from build123d import *

# Parameters (mm, degrees)
F1_DEPTH = 130
F3_DEPTH = 600


with BuildPart() as f1:
    # F0 (on Front) → F1 (new body, symmetric)
    with BuildSketch(Plane.XZ):
        with BuildLine():
            Line((-250.1273464697, -45), (-246.1273464697, -45))
            Line((-246.1273464697, -45), (-246.1273464697, 0))
            ThreePointArc((-246.1273464697, 0), (-241.7339481875, 10.6066017178), (-231.1273464697, 15))
            Line((-231.1273464697, 15), (298.8726535303, 15))
            ThreePointArc((298.8726535303, 15), (309.4792552481, 10.6066017178), (313.8726535303, 0))
            Line((313.8726535303, 0), (313.8726535303, -45))
            Line((313.8726535303, -45), (317.8726535303, -45))
            Line((317.8726535303, -45), (317.8726535303, 0))
            ThreePointArc((317.8726535303, 0), (312.3076823729, 13.4350288425), (298.8726535303, 19))
            Line((298.8726535303, 19), (-231.1273464697, 19))
            ThreePointArc((-231.1273464697, 19), (-244.5623753122, 13.4350288425), (-250.1273464697, 0))
            Line((-250.1273464697, 0), (-250.1273464697, -45))
        make_face()
    extrude(amount=F1_DEPTH, both=True)

    # F2 (on face) → F3 (cut)
    with BuildSketch(Plane.YZ.offset(317.8726535303)):
        with BuildLine():
            Line((-70, -45), (70, -45))
            Line((70, -45), (70, -40))
            ThreePointArc((70, -40), (68.5355339059, -36.4644660941), (65, -35))
            Line((65, -35), (-65, -35))
            ThreePointArc((-65, -35), (-68.5355339059, -36.4644660941), (-70, -40))
            Line((-70, -40), (-70, -45))
        make_face()
    extrude(amount=-F3_DEPTH, mode=Mode.SUBTRACT)


solid = f1.part
Read the model definition and answer for the solid it produces. Units are mm, in the model's axes. A direction names the side the tool comes from. Round coordinates to 2 decimals unless told otherwise and drop trailing zeros. Loops run counter-clockwise (first coordinate to the right, second up) from the corner with the lowest first, then second, coordinate; pieces in that order, holes last. Notation, with made-up numbers: (-16.75, 88) - (28.25, 88) arc R9 cw to (28.25, 97) - close; hole circle Ø2 at (85.25, -10). An arc over 180 degrees is marked (long way). One line per question, with ' | ' between items. Start each with the question number.
Q1. Flat-ended cylindrical pins translate along their axes: pin 1 (3 mm diameter, centred on x = 316, y = -19, fed in from -Z); pin 2 (3 mm diameter, centred on x = 192.5, y = -14, fed in from -Z). Find the tip coordinate at first contact, or state that the pin passes through.
Q2. Section A-A on z = -10 is taken. Give the vertices of the cut face in (x, y), plus the area to 3 significant figures.
Q3. Section B-B on y = 54 is taken. Give the vertices of the cut face in (x, z).
Q4. For a pull along X with two mould halves and no side action, classify faces 1 (the flat face through (-246.127, -2, -23)), 2 (the cylindrical face through (312.45, -1.82, 13.29)), 3 (the cylindrical face through (-244.414, -1.82, 13.582)) as +X half, -X half, draft (parallel to the pull), parting line (faces both ways), or undercut.
Q5. For faces 4 (the cylindrical face through (309.362, -1.82, 10.723)), 5 (the flat face through (33, -130, 16)), determine the directions among +Z, -Z, +X, -X, +Y, -Y from which every point of the face is accessible in a straight line to the end or side of a thin tool.
Q6. Section C-C on x = -31 is taken. Give the vertices of the cut face in (y, z).
Q7. Find the intervals of material crossed by L1, parallel to X at y = 104, z = -6.5; L2, parallel to Z at x = -169, y = 77.5; L3, parallel to X at y = 57, z = 12.5, in increasing order.
Q8. Section D-D on y = -104.5 is taken. Give the vertices of the cut face in (x, z).
Established:
1) pin 1: z = -35 | pin 2: z = 15
2) outline: (-250.13, -130) - (-246.13, -130) - (-246.13, 130) - (-250.13, 130) - close; (313.87, -130) - (317.87, -130) - (317.87, 130) - (313.87, 130) - close | area: 2,080 mm²
3) outline: (-250.13, -35) - (-246.13, -35) - (-246.13, 0) arc R15 cw to (-231.13, 15) - (298.87, 15) arc R15 cw to (313.87, 0) - (313.87, -35) - (317.87, -35) - (317.87, 0) arc R19 ccw to (298.87, 19) - (-231.13, 19) arc R19 ccw to (-250.13, 0) - close
4) face 1: undercut | face 2: +X half | face 3: -X half
5) face 4: -Z, +Y, -Y | face 5: +Z, -Z, +X, -X, -Y
6) outline: (-130, 15) - (130, 15) - (130, 19) - (-130, 19) - close
7) L1: -250.13 to -246.13, 313.87 to 317.87 | L2: 15 to 19 | L3: -245.44 to -239.42, 307.16 to 313.18
8) outline: (-250.13, -45) - (-246.13, -45) - (-246.13, 0) arc R15 cw to (-231.13, 15) - (298.87, 15) arc R15 cw to (313.87, 0) - (313.87, -45) - (317.87, -45) - (317.87, 0) arc R19 ccw to (298.87, 19) - (-231.13, 19) arc R19 ccw to (-250.13, 0) - close
